from build123d import *

# Parameters (mm, degrees)
CHAMFER1_SIZE = 0.762
FILLET2_R     = 1.524
FILLET3_R     = 0.762


with BuildPart() as part:
    # Sketch1 → Revolve1 (revolve)
    with BuildSketch(Plane.XY, mode=Mode.PRIVATE) as revolve1_sk:
        with BuildLine():
            Line((0, 0), (-9.525, 0))
            Line((-9.525, 0), (-9.525, 3.175))
            Line((-9.525, 3.175), (-8.001, 3.175))
            Line((-8.001, 3.175), (-8.001, 4.699))
            Line((-8.001, 4.699), (-6.477, 4.699))
            Line((-6.477, 4.699), (-3.175, 19.05))
            Line((-3.175, 19.05), (-4.7752, 19.05))
            Line((-4.7752, 19.05), (-4.7752, 20.574))
            Line((-4.7752, 20.574), (-3.49192268, 20.574))
            ThreePointArc((-3.49192268, 20.574), (-4.364903349, 25.7175), (0, 28.575))
            Line((0, 28.575), (0, 0))
        make_face()
    revolve(revolve1_sk.sketch.rotate(Axis((0, 0, 0), (0, 1, 0)), 270), axis=Axis((0, 0, 0), (0, 1, 0)))

    # Chamfer1
    chamfer1_edges = [part.edges().sort_by_distance(p)[0] for p in [
        (0, 3.175, 9.525),
    ]]
    chamfer(chamfer1_edges, length=CHAMFER1_SIZE)

    # Fillet2
    fillet2_edges = [part.edges().sort_by_distance(p)[0] for p in [
        (0, 4.699, 8.001),
    ]]
    fillet(fillet2_edges, radius=FILLET2_R - 0.0001)  # a hair under: the kernel refuses the full size

    # Fillet3
    fillet3_edges = [part.edges().sort_by_distance(p)[0] for p in [
        (0, 19.05, 4.7752),
        (0, 20.574, 4.7752),
    ]]
    fillet(fillet3_edges, radius=FILLET3_R - 0.0001)  # a hair under: the kernel refuses the full size


solid = part.part
Work out the finished part from the listing and answer in its coordinate system (mm). A direction names the side the tool comes from. Coordinates: 2 decimals unless noted, no trailing zeros. Loops run counter-clockwise (first coordinate to the right, second up) from the corner with the lowest first, then second, coordinate; pieces in that order, holes last. Notation, with made-up numbers: M -2.75,6.25 L 10.25,6.25 A18 cw 10.25,39.25 Z; hole C 0.25,-16 d8. An arc over 180 degrees is marked long. Answer in a Markdown table with one row per item. Add a question column.
1. Consider L1, parallel to Y at x = 4.75, z = -4.5; L2, parallel to Y at x = -4, z = 7.25 (3 decimals); L3, parallel to X at y = 8.5, z = -4. Determine where each line is inside the solid, lowest interval first.
2. A tool of negligible diameter and unlimited length cuts with its end or side. For faces 4 (the conical face through (2.7, 13.57, 3.52)), 5 (the cylindrical face through (5.796, 1.223, 7.559)), from which of +Z, -Z, +X, -X, +Y, -Y can it reach the whole face along a straight path? Write none if from no direction.
3. The mould has two halves that part along Y. Classify faces 1 (the flat face through (0, 0, 0)), 2 (the flat face through (2, 19.05, 3)), 3 (the flat face through (3, 3.175, -8)): pulls with the +Y half, pulls with the -Y half, needs draft (parallel to the pull), parting line crosses it, or undercut.
4. Flat-ended cylindrical pins translate along their axes: P1, Ø6, axis at x = 7.5, y = 4.5, coming from the +Z side; P2, Ø2, axis at x = -5.5, y = 8.5, coming from the -Z side; P3, Ø5, axis at y = 23.5, z = -2.5, coming from the -X side. Find the tip coordinate at first contact, or state that the pin passes through.
5. Find section D-D, the plane y = 5.75. Write down the section's boundary in (x, z), then the cut area to 3 significant figures.
6. Find section C-C, the plane y = 27.25. Write down the section's boundary in (x, z).
Reported:
| question | item | result |
|---|---|---|
| 1 | L1 | y = 0 to 4.7 |
| 1 | L2 | y = 0 to 3.175 |
| 1 | L3 | x = -3.92 to 3.92 |
| 2 | face 4 | none |
| 2 | face 5 | +Y, -Y |
| 3 | face 1 | pulls with the -Y half |
| 3 | face 2 | undercut |
| 3 | face 3 | pulls with the +Y half |
| 4 | P1 | stops at z = 7.88 |
| 4 | P2 | stops at z = -3.39 |
| 4 | P3 | stops at x = -4.76 |
| 5 | outline | C 0,0 d12.47 |
| 5 | area | 122 mm^2 |
| 6 | outline | C 0,0 d6.59 |
